from build123d import *
from build123d.topology import SkipClean

# Parameters (mm, degrees)
BOSS_EXTRUDE1_DEPTH       = 48
SKETCH2_W                 = 14
SKETCH2_H                 = 10
BOSS_EXTRUDE2_DEPTH       = 50
CUT_EXTRUDE1_DEPTH        = 98
M8X1_0_TAPPED_HOLE1_D     = 7
M8X1_0_TAPPED_HOLE1_DEPTH = 10
M8X1_0_TAPPED_HOLE1_TIP   = 2.103012167
FILLET1_R                 = 6
SKETCH7_R                 = 38.5
SKETCH7_R_2               = 35
BOSS_EXTRUDE3_DEPTH       = 10
SKETCH8_R                 = 35
CUT_EXTRUDE2_DEPTH        = 90
BOSS_EXTRUDE4_DEPTH       = 5
BOSS_EXTRUDE4_DEPTH_BACK  = 10
SKETCH10_R                = 12
SKETCH10_R_2              = 9
BOSS_EXTRUDE5_START       = 25
SKETCH11_R                = 10
SKETCH11_R_2              = 9
BOSS_EXTRUDE5_DEPTH       = 25
SKETCH12_R                = 9
CUT_EXTRUDE3_DEPTH        = 42
BOSS_EXTRUDE6_DEPTH       = 7.5
BOSS_EXTRUDE7_START       = 7.5
BOSS_EXTRUDE7_DEPTH       = 7.5
BOSS_EXTRUDE8_DEPTH       = 10


with BuildPart() as part:
    # Sketch1 → Boss-Extrude1 (new body)
    with BuildSketch(Plane.XY):
        with BuildLine():
            Line((0, 0), (0, 25.00039893))
            Line((0, 25.00039893), (22, 25.00039893))
            ThreePointArc((22, 25.00039893), (51.667114877, 29.062120939), (80, 38.751440389))
            Line((80, 38.751440389), (80, 6.798665084))
            ThreePointArc((80, 6.798665084), (51.198552391, 1.705464917), (22, 0))
            Line((22, 0), (0, 0))
        make_face()
    extrude(amount=BOSS_EXTRUDE1_DEPTH)

    # Sketch2 → Boss-Extrude2 (add)
    with BuildSketch(Plane.XY.offset(48)):
        with Locations((11.5, 12.5)):
            Rectangle(SKETCH2_W, SKETCH2_H)
    boss_extrude2 = extrude(amount=BOSS_EXTRUDE2_DEPTH)

    # Mirror1: Boss-Extrude2 across plane
    add(boss_extrude2.mirror(Plane.XY.offset(24)))

    # Sketch3 → Cut-Extrude1 (cut)
    with BuildSketch(Plane(origin=(0, 0, 0), x_dir=(1, 0, 0), z_dir=(0, 1, 0))):
        Polygon((32.759036304, 13.5), (11.5, 13.5), (-23.123003772, 13.5), (-23.123003772, 84.867154232), (32.759036304, 84.867154232), align=None)
    extrude(amount=CUT_EXTRUDE1_DEPTH, mode=Mode.SUBTRACT)

    # M8x1.0 Tapped Hole1
    with Locations(Plane(origin=(11.5, 17.5, 86), x_dir=(0, 0, 1), z_dir=(0, 1, 0))):
        with Locations((0, 0)):
            Hole(M8X1_0_TAPPED_HOLE1_D / 2, depth=M8X1_0_TAPPED_HOLE1_DEPTH)
            with Locations((0, 0, -(M8X1_0_TAPPED_HOLE1_DEPTH + M8X1_0_TAPPED_HOLE1_TIP / 2))):  # 118° drill point
                Cone(0, M8X1_0_TAPPED_HOLE1_D / 2, M8X1_0_TAPPED_HOLE1_TIP, mode=Mode.SUBTRACT)

    # Fillet1
    fillet1_edges = [part.edges().sort_by_distance(p)[0] for p in [
        (18.5, 12.5, 98),
        (4.5, 12.5, 98),
    ]]
    fillet(fillet1_edges, radius=FILLET1_R)

    # Sketch7 → Boss-Extrude3 (add)
    with BuildSketch(Plane.ZY.offset(-80)):
        with Locations((24, 60.00039893)):
            Circle(SKETCH7_R)
        with Locations((24, 60.00039893)):
            Circle(SKETCH7_R_2, mode=Mode.SUBTRACT)
    extrude(amount=BOSS_EXTRUDE3_DEPTH)

    # Sketch8 → Cut-Extrude2 (cut)
    with BuildSketch(Plane.ZY.offset(-80)):
        with Locations(Location((24, 60.00039893, 0), (0, 0, 226.708192407))):
            Circle(SKETCH8_R)
    extrude(amount=CUT_EXTRUDE2_DEPTH, mode=Mode.SUBTRACT)

    # Sketch10 → Boss-Extrude4 (add, two sides: drawn at the far end of the back side and taken through both)
    with BuildSketch(Plane.XZ.offset(-BOSS_EXTRUDE4_DEPTH_BACK)):
        with Locations((14.5, 24)):
            Circle(SKETCH10_R)
        with Locations((14.5, 24)):
            Circle(SKETCH10_R_2, mode=Mode.SUBTRACT)
    extrude(amount=BOSS_EXTRUDE4_DEPTH + BOSS_EXTRUDE4_DEPTH_BACK)

    # Sketch11 → Boss-Extrude5 (add)
    with BuildSketch(Plane.XZ.offset(5).offset(BOSS_EXTRUDE5_START)):
        with Locations((14.5, 24)):
            Circle(SKETCH11_R)
        with Locations((14.5, 24)):
            Circle(SKETCH11_R_2, mode=Mode.SUBTRACT)
    extrude(amount=-BOSS_EXTRUDE5_DEPTH)

    # Sketch12 → Cut-Extrude3 (cut)
    with BuildSketch(Plane(origin=(0, 0, 0), x_dir=(-1, 0, 0), z_dir=(0, -1, 0))):
        with Locations(Location((-14.5, -24, 0), (0, 0, 180))):
            Circle(SKETCH12_R)
    extrude(amount=-CUT_EXTRUDE3_DEPTH, mode=Mode.SUBTRACT)

    # Sketch13 → Boss-Extrude6 (add)
    with BuildSketch(Plane.XY.offset(48)):
        with BuildLine():
            Line((0, 25.00039893), (0, 0))
            Line((0, 0), (22, 0))
            ThreePointArc((22, 0), (51.198552391, 1.705464917), (80, 6.798665084))
            Line((80, 6.798665084), (80, 29.896412483))
            Line((80, 29.896412483), (80, 34.524920524))
            Line((80, 34.524920524), (70, 34.524920524))
            Line((70, 34.524920524), (69.729925021, 34.524920524))
            ThreePointArc((69.729925021, 34.524920524), (46.24106465, 27.877911315), (22, 25.00039893))
            Line((22, 25.00039893), (0, 25.00039893))
        make_face()
    extrude(amount=BOSS_EXTRUDE6_DEPTH)

    # Sketch14 → Boss-Extrude7 (add)
    with BuildSketch(Plane(origin=(0, 0, 0), x_dir=(-1, 0, 0), z_dir=(0, 0, -1)).offset(BOSS_EXTRUDE7_START)):
        with BuildLine():
            Line((-80, 29.896412483), (-80, 6.798665084))
            ThreePointArc((-80, 6.798665084), (-51.198552391, 1.705464917), (-22, 0))
            Line((-22, 0), (0, 0))
            Line((0, 0), (0, 25.00039893))
            Line((0, 25.00039893), (-22, 25.00039893))
            ThreePointArc((-22, 25.00039893), (-46.24106465, 27.877911315), (-69.729925021, 34.524920524))
            Line((-69.729925021, 34.524920524), (-70, 34.524920524))
            Line((-70, 34.524920524), (-80, 34.524920524))
            Line((-80, 34.524920524), (-80, 29.896412483))
        make_face()
    extrude(amount=-BOSS_EXTRUDE7_DEPTH)

    # Sketch15 → Boss-Extrude8 (add)
    with SkipClean():  # the faces are left unmerged after this step: merging them gives an invalid solid
        with BuildSketch(Plane(origin=(80, 0, 0), x_dir=(0, 0, -1), z_dir=(1, 0, 0))):
            with BuildLine():
                Line((-55.5, 6.798665084), (-55.5, 44.744252628))
                ThreePointArc((-55.5, 44.744252628), (-24, 25.00039893), (7.5, 44.744252628))
                Line((7.5, 44.744252628), (7.5, 6.798665084))
                Line((7.5, 6.798665084), (-55.5, 6.798665084))
            make_face()
            with BuildLine():
                Line((-55.5, 506.798665084), (7.5, 506.798665084))
                Line((7.5, 506.798665084), (7.5, 75.256545232))
                ThreePointArc((7.5, 75.256545232), (-24, 95.00039893), (-55.5, 75.256545232))
                Line((-55.5, 75.256545232), (-55.5, 506.798665084))
            make_face()
        extrude(amount=-BOSS_EXTRUDE8_DEPTH)


solid = part.part
Model file for the job. Use its own axes, mm. A direction names the side the tool comes from. Coordinates: 2 decimals unless noted, no trailing zeros. Write each loop counter-clockwise with the first axis right and the second up, starting at its lowest first coordinate (ties: lowest second). Pieces come first, ordered by that corner, then holes. Notation, with made-up numbers: (62.5, 20) -> (107.5, 20) arc R19 ccw to (107.5, 30) -> close; hole circle Ø10 at (20, 57.25). An arc over 180 degrees is marked (long way). One line per item, written item: value. Start each with the question number.
1) Which spindle directions (+Z, -Z, +X, -X, +Y, -Y) get a long thin tool onto all of the face, cutting with end or side? Do faces 1 (the face through (11, 7.5, 76)), 2 (the face through (11, 17.5, 76)), 3 (the face through (4, 25, 24)), 4 (the face through (12, -5, 34)). Say none if no direction does.
2) Slice it at D-D on z = 77. Write the cut outline in (x, y), then the cut area to 3 significant figures.
3) Probe probe 1 along X at (y, z) = (13, 86); probe 2 along X at (y, z) = (8, 24); probe 3 along Z at (x, y) = (14, -11). List the from-to ranges inside material, lowest first.
4) Flat gauge pins, fed straight in: pin 1 Ø1 at (x, z) = (24, 14) entering from -Y; pin 2 Ø4 at (x, z) = (53.5, 21.5) entering from +Y; pin 3 Ø10 at (x, z) = (20, 47.5) entering from +Y; pin 4 Ø12 at (x, z) = (13.5, 26) entering from -Y. Where does each tip first touch, or does it go through?
5) Slice it at C-C on y = 445. Write the cut outline in (x, z), then the cut area to 3 significant figures.
6) Pull direction X, two halves, no side cores. Call faces 5 (the face through (23.084, -2.857, 26.703)), 6 (the face through (51.605, 1.753, 23.559)), 7 (the face through (75, 297, -7.5)), 8 (the face through (4.5, 12, 73)): +X half, -X half, draft (parallel to the pull), parting line (faces both ways), or undercut.
7) Slice it at B-B on x = 63. Write the cut outline in (y, z), then the cut area to 3 significant figures.
8) Slice it at A-A on z = 6. Write the cut outline in (x, y).
Answers follow:
1. face 1: +Z, +X, -X, -Y
1. face 2: +Z, +X, -X, +Y
1. face 3: +Z, -Z, -X, +Y
1. face 4: -Y
2. outline: (4.5, 7.5) -> (18.5, 7.5) -> (18.5, 17.5) -> (4.5, 17.5) -> close
2. area: 140 mm2
3. probe 1: 4.5 to 8, 15 to 18.5
3. probe 2: 0 to 5.5, 23.5 to 80
3. probe 3: 14.01 to 15.01, 32.99 to 33.99
4. pin 1: y = 0
4. pin 2: y = 25.29
4. pin 3: y = 25.15
4. pin 4: through
5. outline: (70, -7.5) -> (80, -7.5) -> (80, 55.5) -> (70, 55.5) -> close
5. area: 630 mm2
6. face 5: undercut
6. face 6: +X half
6. face 7: draft
6. face 8: -X half
7. outline: (3.37, -7.5) -> (32.21, -7.5) -> (32.21, 2.73) arc R35 cw to (32.21, 45.27) -> (32.21, 55.5) -> (3.37, 55.5) -> close
7. area: 1,610 mm2
8. outline: (0, 0) -> (22, 0) arc R250.8 ccw to (80, 6.8) -> (80, 29.98) -> (55.35, 29.98) arc R155.03 cw to (22, 25) -> (0, 25) -> close; (70, 90.02) -> (80, 90.02) -> (80, 506.8) -> (70, 506.8) -> close
